Part model, mm, in its own coordinate system. Face numbers are marked on the shaded views. A direction names the side the tool comes from. Round coordinates to 2 decimals unless told otherwise and drop trailing zeros. Loops run counter-clockwise (first coordinate to the right, second up) from the corner with the lowest first, then second, coordinate; pieces in that order, holes last. Notation, with made-up numbers: (-29, -24.75) -> (29, -24.75) arc R11 cw to (29, -16.75) -> close; hole circle Ø6 at (33.25, 74). An arc over 180 degrees is marked (long way). Use a Markdown table: item, result. Add a question column.
Item 1: Cut at D-D, the plane z = 26.5. List the corners of the cut face in (x, y).
Item 2: Probe line 1 (Z direction, x = -5, y = 17.5); line 2 (X direction, y = -18, z = -29); line 3 (Z direction, x = -26, y = 15). List the from-to ranges inside material, lowest first. Write a range as [from, to].
Item 3: Cut at B-B, the plane x = 0. List the corners of the cut face in (y, z), plus the area to 3 significant figures.
Item 4: Cut at C-C, the plane y = 13.5. List the corners of the cut face in (x, z).
Item 5: Two-plate mould, pull along X, no slides. Class the marked faces 6, 7, 8 and 9: pulls with the +X half, pulls with the -X half, needs draft (parallel to the pull), parting line crosses it, or undercut.
Item 6: Flat gauge pins, fed straight in: pin 1 (1 mm diameter, centred on y = -4, z = -1.5, fed in from -X); pin 2 (3 mm diameter, centred on x = 38.5, y = 13, fed in from +Z); pin 3 (1.5 mm diameter, centred on y = -9, z = 24, fed in from -X). Where does each tip first touch, or does it go through?
Item 7: Cut at A-A, the plane z = -3. List the corners of the cut face in (x, y), plus the area to 3 significant figures.
Item 8: Which spindle directions (+Z, -Z, +X, -X, +Y, -Y) get a long thin tool onto all of the face, cutting with end or side? Do the marked faces 1, 2, 3, 4 and 5. Say none if no direction does.
```python
from build123d import *

# Parameters (mm, degrees)
SKETCH_1_W              = 20
SKETCH_1_H              = 40
EXTRUDE_763_DEPTH       = 20
FILLET_1_R              = 10
FILLET_2_R              = 2
CUT_EXTRUDE_1402_REACH  = 104.816
SKETCH_2_R              = 5
HOLE_WIZARD_M2_5_REACH  = 104.816
HOLE_WIZARD_M2_5_BORE_R = 1.025


with BuildPart() as part:
    # Эскиз1 → Extrude 763 (new, symmetric)
    with BuildSketch(Plane(origin=(0, 0, 0), x_dir=(1, 0, 0), z_dir=(0, 1, 0))):
        Polygon((-38.118802154, -50), (38.118802154, -50), (47.483339502, -66.219854476), (52.679491924, -63.219854476), (16.179491924, 0), (33.5, 10), (18.488893001, 36), (-18.488893001, 36), (-33.5, 10), (-16.179491924, 0), (-52.679491924, -63.219854476), (-47.483339502, -66.219854476), align=None)
        Polygon((-35.809401077, -46), (-19.643593539, -18), (19.643593539, -18), (35.809401077, -46), align=None, mode=Mode.SUBTRACT)
        with Locations((0, 10)):
            Rectangle(SKETCH_1_W, SKETCH_1_H, mode=Mode.SUBTRACT)
    extrude(amount=EXTRUDE_763_DEPTH, both=True)

    # Скругление1
    fillet_1_edges = [part.edges().sort_by_distance(p)[0] for p in [
        (-18.488893001, 0, -36),
        (18.488893001, 0, -36),
        (19.643593539, 0, 18),
        (-19.643593539, 0, 18),
    ]]
    fillet(fillet_1_edges, radius=FILLET_1_R)

    # Скругление2
    fillet_2_edges = [part.edges().sort_by_distance(p)[0] for p in [
        (35.809401077, 0, 46),
        (-35.809401077, 0, 46),
    ]]
    fillet(fillet_2_edges, radius=FILLET_2_R)

    # Cut-Extrude 1402: up to this face of the body (flat: up to its plane)
    cut_extrude_1402_end = Plane(part.part.faces().sort_by_distance((0, 0, 10))[0])
    # Эскиз2 → Cut-Extrude 1402 (cut, up to the picked face)
    with BuildSketch(Plane.XY.offset(50), mode=Mode.PRIVATE) as cut_extrude_1402_sk1:
        with Locations((0, -10)):
            Circle(SKETCH_2_R)
    cut_extrude_1402_tool1 = split(extrude(cut_extrude_1402_sk1.sketch, amount=-CUT_EXTRUDE_1402_REACH, mode=Mode.PRIVATE), bisect_by=cut_extrude_1402_end, keep=Keep.BOTH, mode=Mode.PRIVATE)
    add(cut_extrude_1402_tool1.solids().sort_by(Axis((0, -10, 50), (0, 0, -1)))[0], mode=Mode.SUBTRACT)

    # Заглушка подшипника M2.5 bore → Заглушка подшипника M2.5 (cut, up to next)
    with BuildSketch(Plane.XY.offset(50), mode=Mode.PRIVATE) as hole_wizard_m2_5_sk1:
        with Locations((-10, -10)):
            Circle(HOLE_WIZARD_M2_5_BORE_R)
    hole_wizard_m2_5_tool1 = extrude(hole_wizard_m2_5_sk1.sketch, amount=-HOLE_WIZARD_M2_5_REACH, mode=Mode.PRIVATE) & part.part
    # Заглушка подшипника M2.5 bore → Заглушка подшипника M2.5 (cut, up to next)
    with BuildSketch(Plane.XY.offset(50), mode=Mode.PRIVATE) as hole_wizard_m2_5_sk2:
        with Locations((10, -10)):
            Circle(HOLE_WIZARD_M2_5_BORE_R)
    hole_wizard_m2_5_tool2 = extrude(hole_wizard_m2_5_sk2.sketch, amount=-HOLE_WIZARD_M2_5_REACH, mode=Mode.PRIVATE) & part.part
    add(hole_wizard_m2_5_tool1.solids().sort_by_distance((-10, -10, 50))[0], mode=Mode.SUBTRACT)
    add(hole_wizard_m2_5_tool2.solids().sort_by_distance((10, -10, 50))[0], mode=Mode.SUBTRACT)


solid = part.part
```
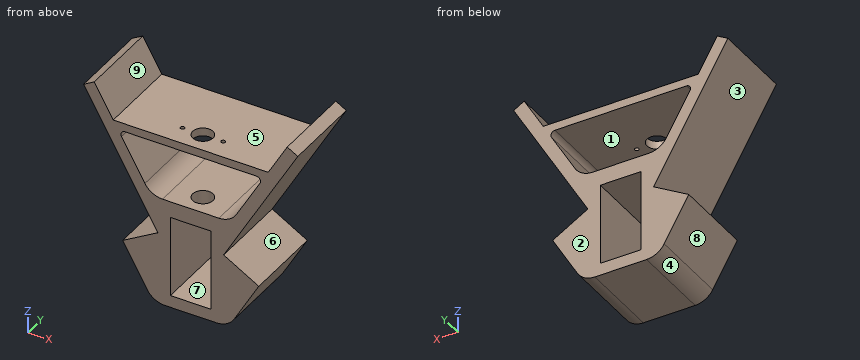
A:
| question | item | result |
|---|---|---|
| 1 | outline | (-31.48, -20) -> (-24.55, -20) -> (-24.55, 20) -> (-31.48, 20) -> close; (24.55, -20) -> (31.48, -20) -> (31.48, 20) -> (24.55, 20) -> close |
| 2 | line 1 | z = [-36, -30], [10, 18], [46, 50] |
| 2 | line 2 | x = [-22.53, -10], [10, 22.53] |
| 2 | line 3 | z = [-22.99, -5.67], [17.01, 29.01], [46, 50] |
| 3 | outline | (-20, -36) -> (20, -36) -> (20, -30) -> (-20, -30) -> close; (-20, 10) -> (-15, 10) -> (-15, 18) -> (-20, 18) -> close; (-20, 46) -> (-15, 46) -> (-15, 50) -> (-20, 50) -> close; (-5, 10) -> (20, 10) -> (20, 18) -> (-5, 18) -> close; (-5, 46) -> (20, 46) -> (20, 50) -> (-5, 50) -> close |
| 3 | area | 600 mm^2 |
| 4 | outline | (-52.68, 63.22) -> (-16.18, 0) -> (-33.5, -10) -> (-21.38, -31) arc R10 ccw to (-12.72, -36) -> (12.72, -36) arc R10 ccw to (21.38, -31) -> (33.5, -10) -> (16.18, 0) -> (52.68, 63.22) -> (47.48, 66.22) -> (38.12, 50) -> (-38.12, 50) -> (-47.48, 66.22) -> close; hole (-34.08, 43) -> (-22.53, 23) arc R10 ccw to (-13.87, 18) -> (13.87, 18) arc R10 ccw to (22.53, 23) -> (34.08, 43) arc R2 ccw to (32.35, 46) -> (-32.35, 46) arc R2 ccw to start; hole (-10, -30) -> (10, -30) -> (10, 10) -> (-10, 10) -> close |
| 5 | face 6 | pulls with the +X half |
| 5 | face 7 | undercut |
| 5 | face 8 | pulls with the -X half |
| 5 | face 9 | undercut |
| 6 | pin 1 | stops at x = -19.64 |
| 6 | pin 2 | stops at z = 53.26 |
| 6 | pin 3 | stops at x = -30.47 |
| 7 | outline | (-21.38, -20) -> (-10, -20) -> (-10, 20) -> (-21.38, 20) -> close; (10, -20) -> (21.38, -20) -> (21.38, 20) -> (10, 20) -> close |
| 7 | area | 910 mm^2 |
| 8 | face 1 | +Y, -Y |
| 8 | face 2 | +Z, -Z, +X, -X, +Y |
| 8 | face 3 | -X, +Y, -Y |
| 8 | face 4 | -Z, -X, +Y, -Y |
| 8 | face 5 | +Z, +Y, -Y |
